from build123d import *

# Parameters (mm, degrees)
F1_DEPTH = 18
F2_SIZE  = 5


with BuildPart() as f1:
    # F0 (on Front) → F1 (new body)
    with BuildSketch(Plane.XZ):
        Polygon((-58, 80), (-58, 0), (-9, 0), (-9, 40), (9, 40), (9, 0), (58, 0), (58, 80), align=None)
    extrude(amount=F1_DEPTH)

    # F2
    f2_edges = [f1.edges().sort_by_distance(p)[0] for p in [
        (-58, -9, 80),
        (-58, -9, 0),
        (58, -9, 80),
        (58, -9, 0),
    ]]
    chamfer(f2_edges, length=F2_SIZE)


solid = f1.part
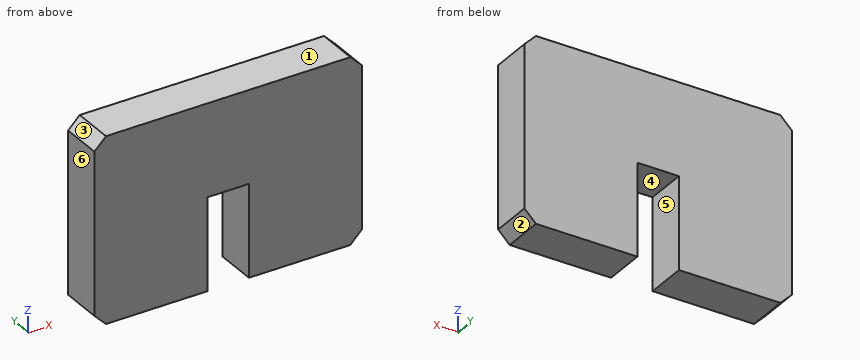
Source: CAD feature listing. Evaluate the final solid. Frame: model axes, mm. Face numbers are marked on the shaded views. A direction names the side the tool comes from. Give positions to 0.01 mm unless a question says otherwise; leave off trailing zeros. Loops run counter-clockwise (first coordinate to the right, second up) from the corner with the lowest first, then second, coordinate; pieces in that order, holes last. Notation, with made-up numbers: (40.25, 6) -> (81.25, 6) arc R20 cw to (81.25, 22) -> close; hole circle Ø6 at (58, -25.75). An arc over 180 degrees is marked (long way). Use a Markdown table: item, result. Add a question column.
1) First-contact query: pin 1 (9 mm diameter, centred on x = -2.5, y = -9.5, fed in from -Z). Flat tip, straight axial feed; report the tip coordinate or a pass-through.
2) Reachability of the marked faces 5 and 6 from +Z, -Z, +X, -X, +Y, -Y: full face, straight path, thin tool, end or side. Return the list, or none.
3) Section query B-B, the plane y = -15.25. Return the cut outline in (x, z), then the cut area to 3 significant figures.
4) Line query: line 1 along X through (y, z) = (-17, 12); line 2 along Z through (x, y) = (-5, -11); line 3 along X through (y, z) = (-11.75, 4). Output: solid intervals per line, ascending. Write a range as [from, to].
5) Pull-direction query (X, two-part tool) for the marked faces 1, 2, 3 and 4; classes: +X half, -X half, draft (parallel to the pull), parting line (faces both ways), or undercut.
6) Section query A-A, the plane z = 10.5. Return the cut outline in (x, y).
Numbers:
| question | item | result |
|---|---|---|
| 1 | pin 1 | stops at z = 40 |
| 2 | face 5 | -Z, +Y, -Y |
| 2 | face 6 | +Z, -Z, -X, +Y, -Y |
| 3 | outline | (-58, 5) -> (-53, 0) -> (-9, 0) -> (-9, 40) -> (9, 40) -> (9, 0) -> (53, 0) -> (58, 5) -> (58, 75) -> (53, 80) -> (-53, 80) -> (-58, 75) -> close |
| 3 | area | 8,510 mm2 |
| 4 | line 1 | x = [-58, -9], [9, 58] |
| 4 | line 2 | z = [40, 80] |
| 4 | line 3 | x = [-57, -9], [9, 57] |
| 5 | face 1 | draft |
| 5 | face 2 | +X half |
| 5 | face 3 | -X half |
| 5 | face 4 | undercut |
| 6 | outline | (-58, -18) -> (-9, -18) -> (-9, 0) -> (-58, 0) -> close; (9, -18) -> (58, -18) -> (58, 0) -> (9, 0) -> close |
